```python
from build123d import *

# Parameters (mm, degrees)
F0_W     = 100
F0_H     = 25
F1_DEPTH = 3
F2_R     = 5
F3_R     = 3.25
F4_DEPTH = 25


with BuildPart() as f1:
    # F0 (on Front) → F1 (new body)
    with BuildSketch(Plane.XZ):
        Rectangle(F0_W, F0_H)
    extrude(amount=F1_DEPTH)

    # F2
    f2_edges = [f1.edges().sort_by_distance(p)[0] for p in [
        (50, -1.5, 12.5),
        (50, -1.5, -12.5),
        (-50, -1.5, -12.5),
        (-50, -1.5, 12.5),
    ]]
    fillet(f2_edges, radius=F2_R)

    # F3 (on Front) → F4 (cut)
    with BuildSketch(Plane.XZ):
        with BuildLine():
            Line((35.75, -17.689867), (35.75, 0))
            ThreePointArc((35.75, 0), (32.5, 3.25), (29.25, 0))
            Line((29.25, 0), (29.25, -17.689867))
            Line((29.25, -17.689867), (35.75, -17.689867))
        make_face()
        with Locations((-32.5, 0)):
            Circle(F3_R)
    extrude(amount=F4_DEPTH, mode=Mode.SUBTRACT)


solid = f1.part
```
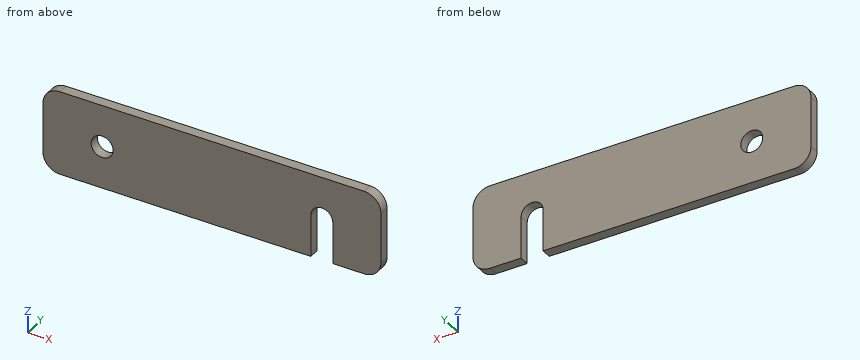
Input: part model. Units: mm. Frame: model coordinates. Give positions to 0.01 mm unless a question says otherwise; leave off trailing zeros. Order: outer loops, then holes, each group sorted by start corner. A loop starts at its lowest first (then second) coordinate and runs counter-clockwise, first axis right, second up.
1. Pin query (flat end, axial travel): pin 1 (6 mm diameter, centred on x = -9, z = 1, fed in from +Y); pin 2 (1 mm diameter, centred on x = 31.5, y = -2, fed in from -Z). Return the tip coordinate at first contact, or that it passes through.
Derived:
pin 1: stops at y = 0
pin 2: stops at z = 2.88
2. Section C-C on y = -2.05. Return the cut outline in (x, z), and give its area (3 significant figures).
Derived:
outline: (-50, -7.5) arc R5 ccw to (-45, -12.5) - (29.25, -12.5) - (29.25, 0) arc R3.25 cw to (35.75, 0) - (35.75, -12.5) - (45, -12.5) arc R5 ccw to (50, -7.5) - (50, 7.5) arc R5 ccw to (45, 12.5) - (-45, 12.5) arc R5 ccw to (-50, 7.5) - close; hole circle Ø6.5 at (-32.5, 0)
area: 2,350 mm2
3. Section B-B on z = -4.75. Return the cut outline in (x, y).
Derived:
outline: (-50, -3) - (29.25, -3) - (29.25, 0) - (-50, 0) - close; (35.75, -3) - (50, -3) - (50, 0) - (35.75, 0) - close
4. Material intervals for L1, parallel to Z at x = -32.5, y = -1.5; L2, parallel to X at y = -2.2, z = 1; L3, parallel to Z at x = -31, y = -0.7, sorted ascending.
Derived:
L1: z = -12.5 to -3.25, 3.25 to 12.5
L2: x = -50 to -35.59, -29.41 to 29.41, 35.59 to 50
L3: z = -12.5 to -2.88, 2.88 to 12.5
5. Section A-A on x = -32.5. Return the cut outline in (y, z).
Derived:
outline: (-3, -12.5) - (0, -12.5) - (0, -3.25) - (-3, -3.25) - close; (-3, 3.25) - (0, 3.25) - (0, 12.5) - (-3, 12.5) - close
6. Section D-D on x = 32.5. Return the cut outline in (y, z), and give its area (4 significant figures).
Derived:
outline: (-3, 3.25) - (0, 3.25) - (0, 12.5) - (-3, 12.5) - close
area: 27.75 mm2
